Study the drawing (mm; zero at the part's minimum x, y, z) and answer. Give positions to 0.01 mm unless a question says otherwise; leave off trailing zeros. Order: outer loops, then holes, each group sorted by start corner. A loop starts at its lowest first (then second) coordinate and runs counter-clockwise, first axis right, second up. Notation, with made-up numbers: (34, 25.5) - (87, 25.5) arc R25 cw to (87, 50.5) - close; hole circle Ø6 at (71.5, 4.25). An arc over 180 degrees is marked (long way). Write each question's results on one line, items separated by ' | '. Start each with the question number.
Q1. Find section B-B on x = 261.5. Give the vertices of the cut face in (y, z) (1 decimal), and give its area (3 significant figures).
Q2. Find section C-C on y = 2.2. Count the separate pieces of the cut face and the enclosed holes in it, and give its area (3 significant figures).
Q3. Find the intervals of material crossed by line 1 along Z through (x, y) = (152.4, 1.9) (1 decimal); line 2 along X through (y, z) = (2.3, 150.5) (1 decimal); line 3 along Z through (x, y) = (190.5, 1.5), in increasing order. Write a range as from..to.
Q4. A flat-ended cylindrical pin translates along its axis: P1, Ø1, axis at y = 0.5, z = 214, coming from the +X side (1 decimal). Find the tip coordinate at first contact, or state that the pin passes through.
Q5. Find section A-A on z = 152.4. Give the vertices of the cut face in (x, y) (1 decimal), and give its area (3 significant figures).
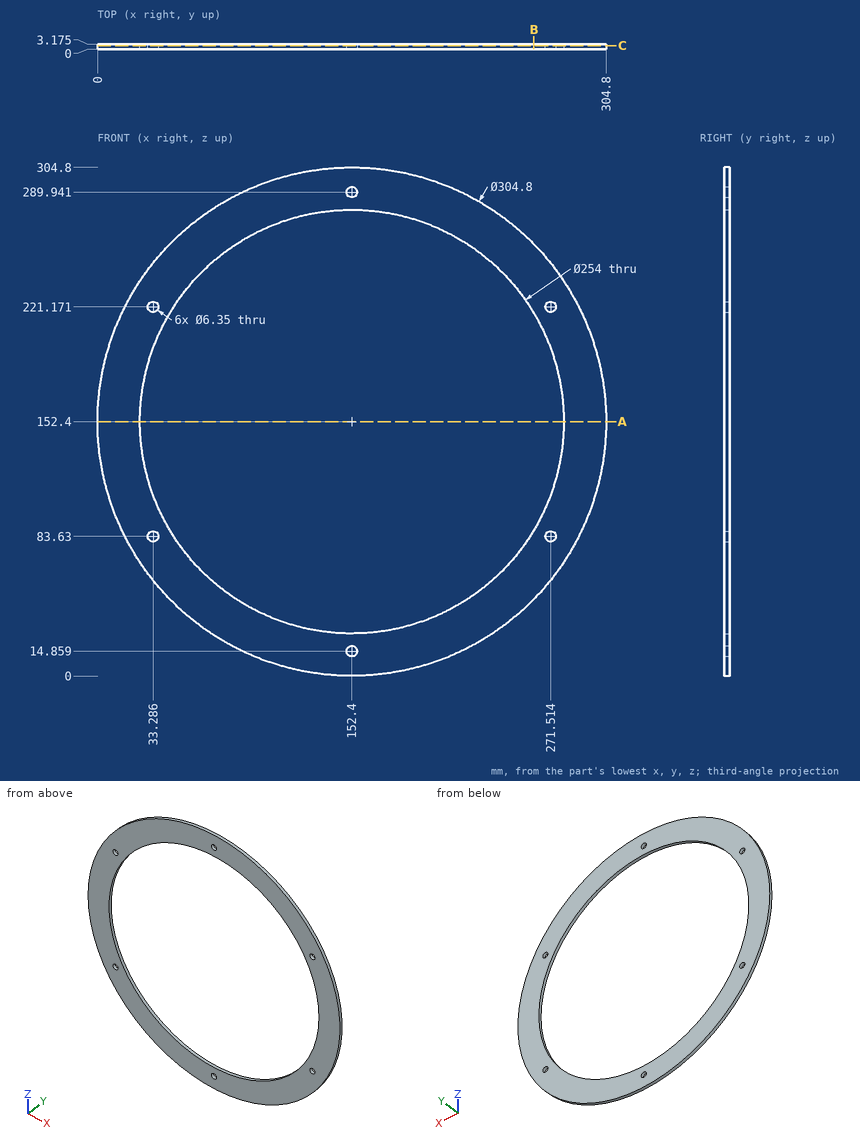
Working result:
1) outline: (0, 46) - (3.2, 46) - (3.2, 87.4) - (0, 87.4) - close; (0, 217.4) - (3.2, 217.4) - (3.2, 258.8) - (0, 258.8) - close | area: 263 mm²
2) separate pieces: 1 | enclosed holes: 7 | area: 22,100 mm²
3) line 1: 0..11.7, 18..25.4, 279.4..286.8, 293.1..304.8 | line 2: 0..25.4, 279.4..304.8 | line 3: 4.84..31.25, 273.55..299.96
4) P1: x = 292
5) outline: (0, 0) - (25.4, 0) - (25.4, 3.2) - (0, 3.2) - close; (279.4, 0) - (304.8, 0) - (304.8, 3.2) - (279.4, 3.2) - close | area: 161 mm²
